Can you work these out from the model? Positions are in its coordinate system, mm. A direction names the side the tool comes from. Give positions to 0.01 mm unless a question says otherwise; leave off trailing zeros. Order: outer loops, then holes, each group sorted by start corner. A loop starts at its lowest first (then second) coordinate and runs counter-clockwise, first axis right, second up. Notation, with made-up numbers: M 9.5,0 L 59.5,0 A17 ccw 59.5,24 Z; hole C 18,58 d8. An arc over 180 degrees is marked long. Use one line per item in the form item = value. Start each with the question number.
1. I need wall thicknesses on L1, parallel to Y at x = 65.5, z = 18; L2, parallel to Z at x = 298.5, y = 7 (3 decimals); L3, parallel to X at y = 5.25, z = 22.5. Which ranges of each line are inside material? Lowest first, please.
2. For faces 1 (the face through (206, 17, 22.225)), 2 (the face through (279.4, 15.38, 23.83)), 3 (the face through (206, 25.4, 13)), which set-ups out of +Z, -Z, +X, -X, +Y, -Y let a thin tool reach every point of the face, with its end or its side?
3. We'd pull the mould along Z, two halves only. Please class faces 4 (the face through (381, 15.1, 1.6)), 5 (the face through (206, 21.916, 13)), 6 (the face through (200, 19, 25.4)), 7 (the face through (200, 19, 0)): +Z half, -Z half, draft (parallel to the pull), parting line (faces both ways), or undercut.
4. I want a section at A-A, the plane z = 14.5. List the corners of the cut face in (x, y) for me, and give its area (3 significant figures).
5. Will this pin go through, and if not, where does the flat tip stop? P1, Ø6, axis at x = 322.5, y = 18.5, coming from the +Z side.
Autodesk Inventor part; units mm, degrees
ref_plane "YZ Plane" through (0, 0, 0) normal (1, 0, 0) x (0, 1, 0)
ref_plane "XZ Plane" through (0, 0, 0) normal (0, 1, 0) x (-1, 0, 0)
ref_plane "XY Plane" through (0, 0, 0) normal (0, 0, 1) x (1, 0, 0)
sketch "Sketch1" plane through (0, 0, 0) normal (0, 0, 1) x (1, 0, 0)
  line L0 (0, 0) -> (406.4, 0)
  line L1 (406.4, 0) -> (406.4, 25.4)
  line L2 (406.4, 25.4) -> (0, 25.4)
  line L3 (0, 25.4) -> (0, 0)
  dimension "d0" = 406.4
  dimension "d1" = 25.4
extrude "Extrusion1" add sketch "Sketch1" along normal blind 25.4
sketch "Sketch2" plane through (406.4, 0, 0) normal (1, 0, 0) x (0, 0, -1)
  line L0 (-22.225, 3.4845) -> (-3.175, 3.4845)
  line L1 (-3.175, 3.4845) -> (-3.175, 21.9155)
  line L2 (-3.175, 21.9155) -> (-22.225, 21.9155)
  line L3 (-22.225, 21.9155) -> (-22.225, 3.4845)
  line L4 (-22.225, 3.4845) -> (-3.175, 21.9155) construction
  line L5 (-3.175, 3.4845) -> (-22.225, 21.9155) construction
  point P0 (-12.7, 12.7)
  dimension "d4" = 19.05
extrude "Extrusion2" cut sketch "Sketch2" against normal blind 406.4
sketch "Sketch3" plane through (0, 0, 25.4) normal (0, 0, 1) x (1, 0, 0)
  arc A0 (31.75, 21.59) -> (31.75, 8.89) centre (31.75, 15.24) ccw
  arc A1 (120.65, 8.89) -> (120.65, 21.59) centre (120.65, 15.24) ccw
  line L0 (31.75, 21.59) -> (120.65, 21.59)
  line L1 (31.75, 8.89) -> (120.65, 8.89)
  arc A2 (158.75, 16.51) -> (158.75, 3.81) centre (158.75, 10.16) ccw
  arc A3 (247.65, 3.81) -> (247.65, 16.51) centre (247.65, 10.16) ccw
  line L2 (158.75, 16.51) -> (247.65, 16.51)
  line L3 (247.65, 3.81) -> (158.75, 3.81)
  line L4 (0, 0) -> (406.4, 0)
  line L5 (406.4, 25.4) -> (0, 25.4)
  line L6 (0, 25.4) -> (0, 0)
  line L7 (25.4, 15.24) -> (25.4, 25.4)
  line L8 (127, 15.24) -> (127, 25.4)
  line L9 (152.4, 10.16) -> (152.4, 0)
  line L10 (254, 10.16) -> (254, 0)
  arc A4 (285.75, 21.59) -> (285.75, 8.89) centre (285.75, 15.24) ccw
  arc A5 (374.65, 8.89) -> (374.65, 21.59) centre (374.65, 15.24) ccw
  line L11 (279.4, 15.24) -> (279.4, 25.4)
  line L12 (285.75, 21.59) -> (374.65, 21.59)
  line L13 (381, 15.24) -> (381, 25.4)
  line L14 (374.65, 8.89) -> (285.75, 8.89)
  line L15 (158.75, 0) -> (158.75, 10.16)
  line L16 (31.75, 15.24) -> (31.75, 25.4)
  line L17 (374.65, 15.24) -> (374.65, 25.4)
  dimension "d7" = 12.7
  dimension "d8" = 12.7
  dimension "d13" = 12.7
  dimension "d14" = 12.7
  dimension "d19" = 101.6
  dimension "d20" = 101.6
  dimension "d22" = 12.7
  dimension "d23" = 12.7
  dimension "d24" = 101.6
  dimension "d25" = 25.4
  dimension "d26" = 25.4
  dimension "d27" = 25.4
  dimension "d28" = 10.16
  dimension "d29" = 10.16
extrude "Extrusion3" cut sketch "Sketch3" against normal blind 25.4 contours L0 A1 L1 A0 | A4 L12 A5 L14 | A2 L2 A3 L3
properties part number "West Coast Side"
Check result:
q1.L1 = 0 to 3.48, 21.92 to 25.4
q1.L2 = 0 to 3.175, 22.225 to 25.4
q1.L3 = 0 to 154.72, 251.68 to 406.4
q2.face_1 = +X, -X
q2.face_2 = +Z, -Z
q2.face_3 = +Z, -Z, +X, -X, +Y
q3.face_4 = draft
q3.face_5 = undercut
q3.face_6 = +Z half
q3.face_7 = -Z half
q4.outline = M 0,0 L 406.4,0 L 406.4,3.48 L 0,3.48 Z; M 0,21.92 L 406.4,21.92 L 406.4,25.4 L 0,25.4 Z
q4.area = 2,830 mm2
q5.P1 = through
